Part model, mm, in its own coordinate system. Round coordinates to 2 decimals unless told otherwise and drop trailing zeros. Loops run counter-clockwise (first coordinate to the right, second up) from the corner with the lowest first, then second, coordinate; pieces in that order, holes last. Notation, with made-up numbers: M -8,19 L 2,19 A10 ccw 2,26 Z; hole C 62,-10.5 d6. An arc over 180 degrees is marked long. Put each result on its own line as item: value. Start each with the question number.
1) Probe line 1 along Y through (x, z) = (1.25, -293.5); line 2 along Y through (x, z) = (-2.75, -273.5). List the from-to ranges inside material, lowest first.
2) Slice it at C-C on z = -305.5. Give the cut face in (x, y).
3) Drop a flat-ended pin along its axis: pin 1 Ø1.9 at (x, z) = (-2, -176) entering from -Y. Give the stop position or say it passes through.
4) Slice it at B-B on y = -8. Give the cut face in (x, z).
Autodesk Inventor part; units mm, degrees
ref_plane "YZ Plane" through (0, 0, 0) normal (1, 0, 0) x (0, 1, 0)
ref_plane "XZ Plane" through (0, 0, 0) normal (0, 1, 0) x (-1, 0, 0)
ref_plane "XY Plane" through (0, 0, 0) normal (0, 0, 1) x (1, 0, 0)
sketch "Sketch1" plane through (0, 0, 0) normal (0, 1, 0) x (-1, 0, 0)
  line L0 (0, 0) -> (0, -180) construction
  line L1 (5, 0) -> (5, -180)
  line L2 (-5, -180) -> (-5, 0)
  arc A0 (5, 0) -> (-5, 0) centre (0, 0) ccw
  arc A1 (-5, -180) -> (5, -180) centre (0, -180) ccw
  circle A2 centre (0, 0) radius 1.65
  line L3 (0, -40) -> (0, -140) construction
  line L4 (1.65, -40) -> (1.65, -140)
  line L5 (-1.65, -140) -> (-1.65, -40)
  arc A3 (1.65, -40) -> (-1.65, -40) centre (0, -40) ccw
  arc A4 (-1.65, -140) -> (1.65, -140) centre (0, -140) ccw
  point P0 (0, -90)
  point P1 (0, -90)
  dimension "d0" = 180
  dimension "d1" = 10
  dimension "d2" = 3.3
  dimension "d3" = 40
  dimension "d5" = 140
  dimension "d6" = 3.3
extrude "Extrusion1" add sketch "Sketch1" along normal blind 6
sketch "Sketch2" plane through (5, 0, 0) normal (1, 0, 0) x (0, 0, -1)
  line L0 (180, 0) -> (180, 6)
  line L1 (0, 0) -> (180, 0)
  line L2 (180, 0) -> (180, 6)
  line L3 (0, 6) -> (180, 6)
  line L4 (0, 0) -> (0, 6)
  line L5 (180, 0) -> (180, 0)
  line L6 (180, 0) -> (180, 6)
  line L7 (180, 6) -> (180, 6)
  line L8 (180, 0) -> (180, 6)
  line L9 (180, 0) -> (0, 0)
  arc A0 (498.004, -84) -> (180, 0) centre (180, -643.9437) ccw
  line L10 (180, 6) -> (0, 6)
  arc A1 (498.004, -78) -> (180, 6) centre (180, -637.9437) ccw
  line L11 (498.004, -78) -> (498.004, -84)
  line L12 (0, 0) -> (180, 0)
  dimension "d9" = 6
  dimension "d10" = 498.004
  dimension "d11" = 90
extrude "Extrusion2" add sketch "Sketch2" against normal blind 10 contours L0 A1 L11 A0
fillet "Fillet1" radius 2 4 edges at (0, -78, -498.004) (5, -81, -498.004) (-5, -81, -498.004) (0, -84, -498.004)
sketch "Sketch3" plane through (0, 6, 0) normal (0, 1, 0) x (1, 0, 0)
  line L0 (-25.1236, -17.4365) -> (19.1239, -17.4365)
  line L1 (19.1239, -17.4365) -> (19.1239, 173.8027)
  line L2 (19.1239, 173.8027) -> (-25.1236, 173.8027)
  line L3 (-25.1236, 173.8027) -> (-25.1236, -17.4365)
  line L4 (-48.0471, -35.7333) -> (42.457, -35.7333)
  line L5 (42.457, -35.7333) -> (42.457, 337.7497)
  line L6 (42.457, 337.7497) -> (-48.0471, 337.7497)
  line L7 (-48.0471, 337.7497) -> (-48.0471, -35.7333)
  line L8 (-102.0639, -92.3443) -> (98.6132, -92.3443)
  line L9 (98.6132, -92.3443) -> (98.6132, 617.9416)
  line L10 (98.6132, 617.9416) -> (-102.0639, 617.9416)
  line L11 (-102.0639, 617.9416) -> (-102.0639, -92.3443)
  point P0 (0, 0)
extrude "Extrusion3" cut sketch "Sketch3" against normal blind 100
properties part number "Part_8_p2"
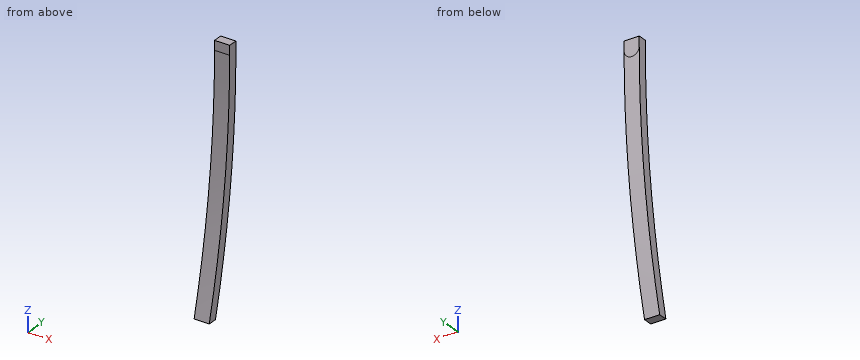
Recorded:
1. line 1: y = -10.08 to -4.08
1. line 2: y = -6.82 to -0.82
2. outline: M -5,-12.35 L 5,-12.35 L 5,-6.35 L -5,-6.35 Z
3. pin 1: stops at y = 0
4. outline: M -5,-313.55 L 5,-313.55 L 5,-281.19 L -5,-281.19 Z
